For this review, take the finished solid that the model builds, in its own axes (mm). A direction names the side the tool comes from. Give positions to 0.01 mm unless a question says otherwise; leave off trailing zeros. Loops run counter-clockwise (first coordinate to the right, second up) from the corner with the lowest first, then second, coordinate; pieces in that order, holes last. Notation, with made-up numbers: (3, -32) - (15, -32) arc R34 cw to (15, 1) - close; hole circle Ø11 at (49.25, 36.5). An arc over 180 degrees is marked (long way). Put each result on its own line as item: value.
from build123d import *

# Parameters (mm, degrees)
SKETCH1_W                = 60
SKETCH1_H                = 21
BOSS_EXTRUDE1_DEPTH      = 10
BOSS_EXTRUDE1_DEPTH_BACK = 10
FILLET1_R                = 6
SKETCH2_R                = 2.2
CUT_EXTRUDE1_DEPTH       = 21
CUT_EXTRUDE2_DEPTH       = 22


with BuildPart() as part:
    # Sketch1 → Boss-Extrude1 (new body, two sides)
    with BuildSketch(Plane.XY) as boss_extrude1_sk:
        Rectangle(SKETCH1_W, SKETCH1_H)
    extrude(amount=BOSS_EXTRUDE1_DEPTH)
    extrude(boss_extrude1_sk.sketch, amount=-BOSS_EXTRUDE1_DEPTH_BACK)

    # Fillet1
    fillet1_edges = [part.edges().sort_by_distance(p)[0] for p in [
        (30, -10.5, 0),
        (-30, -10.5, 0),
        (-30, 10.5, 0),
        (30, 10.5, 0),
    ]]
    fillet(fillet1_edges, radius=FILLET1_R)

    # Sketch2 → Cut-Extrude1 (cut, through all)
    with BuildSketch(Plane.XY.offset(10)):
        with Locations((-24, 5.5)):
            Circle(SKETCH2_R)
        with Locations((24, 5.5)):
            Circle(SKETCH2_R)
        with Locations((24, -5.5)):
            Circle(SKETCH2_R)
        with Locations((-24, -5.5)):
            Circle(SKETCH2_R)
    extrude(amount=-CUT_EXTRUDE1_DEPTH, mode=Mode.SUBTRACT)

    # Sketch3 → Cut-Extrude2 (cut, through all)
    with BuildSketch(Plane(origin=(0, 10.5, 0), x_dir=(1, 0, 0), z_dir=(0, 1, 0))):
        with BuildLine():
            Line((9, -4.5), (-9, -4.5))
            ThreePointArc((-9, -4.5), (-10.414213562, -3.914213562), (-11, -2.5))
            Line((-11, -2.5), (-11, 2.5))
            ThreePointArc((-11, 2.5), (-10.414213562, 3.914213562), (-9, 4.5))
            Line((-9, 4.5), (9, 4.5))
            ThreePointArc((9, 4.5), (10.414213562, 3.914213562), (11, 2.5))
            Line((11, 2.5), (11, -2.5))
            ThreePointArc((11, -2.5), (10.414213562, -3.914213562), (9, -4.5))
        make_face()
    extrude(amount=-CUT_EXTRUDE2_DEPTH, mode=Mode.SUBTRACT)


solid = part.part
1) Take a section at C-C on z = 8.75. State the section outline as (x, y) points, and give its area (3 significant figures).
Geometry check:
outline: (-30, -4.5) arc R6 ccw to (-24, -10.5) - (24, -10.5) arc R6 ccw to (30, -4.5) - (30, 4.5) arc R6 ccw to (24, 10.5) - (-24, 10.5) arc R6 ccw to (-30, 4.5) - close; hole circle Ø4.4 at (-24, -5.5); hole circle Ø4.4 at (-24, 5.5); hole circle Ø4.4 at (24, -5.5); hole circle Ø4.4 at (24, 5.5)
area: 1,170 mm²
2) Wall thickness on line 1 (Y direction, x = -24, z = 0.75); line 2 (X direction, y = 3.25, z = -2); line 3 (Z direction, x = -0.5, y = -6): over which ranges is each line inside the solid? List them lowest first.
Geometry check:
line 1: y = -10.5 to -7.7, -3.3 to 3.3, 7.7 to 10.5
line 2: x = -30 to -11, 11 to 30
line 3: z = -10 to -4.5, 4.5 to 10
3) Take a section at B-B on y = -5.5. State the section outline as (x, z) points, and give its area (3 significant figures).
Geometry check:
outline: (-29.92, -10) - (-26.2, -10) - (-26.2, 10) - (-29.92, 10) - close; (-21.8, -10) - (21.8, -10) - (21.8, 10) - (-21.8, 10) - close; (26.2, -10) - (29.92, -10) - (29.92, 10) - (26.2, 10) - close; hole (-11, -2.5) arc R2 ccw to (-9, -4.5) - (9, -4.5) arc R2 ccw to (11, -2.5) - (11, 2.5) arc R2 ccw to (9, 4.5) - (-9, 4.5) arc R2 ccw to (-11, 2.5) - close
area: 826 mm²
4) Take a section at D-D on y = -8.75. State the section outline as (x, z) points, and give its area (3 significant figures).
Geometry check:
outline: (-28.24, -10) - (28.24, -10) - (28.24, 10) - (-28.24, 10) - close; hole (-11, -2.5) arc R2 ccw to (-9, -4.5) - (9, -4.5) arc R2 ccw to (11, -2.5) - (11, 2.5) arc R2 ccw to (9, 4.5) - (-9, 4.5) arc R2 ccw to (-11, 2.5) - close
area: 935 mm²
5) For faces 1 (the face through (11, 0, 0)), 2 (the face through (0, 10.5, 5)), list the 3-axis set-ups (+Z, -Z, +X, -X, +Y, -Y) from which the entire face can be reached by the end or side of a thin tool; tool diameter is ignored.
Geometry check:
face 1: +Y, -Y
face 2: +Z, -Z, +X, -X, +Y
6) Take a section at A-A on z = 0.75. State the section outline as (x, y) points.
Geometry check:
outline: (-30, -4.5) arc R6 ccw to (-24, -10.5) - (-11, -10.5) - (-11, 10.5) - (-24, 10.5) arc R6 ccw to (-30, 4.5) - close; (11, -10.5) - (24, -10.5) arc R6 ccw to (30, -4.5) - (30, 4.5) arc R6 ccw to (24, 10.5) - (11, 10.5) - close; hole circle Ø4.4 at (-24, -5.5); hole circle Ø4.4 at (-24, 5.5); hole circle Ø4.4 at (24, -5.5); hole circle Ø4.4 at (24, 5.5)
7) Draft analysis for pull direction Z (two halves, no side actions). For faces 3 (the face through (10.4, 0.15, -3.93)), 4 (the face through (0, 0, 10)), 5 (the face through (28.289, -8.696, 0.14)), state which applies: pulls with the +Z half, pulls with the -Z half, needs draft (parallel to the pull), parting line crosses it, or undercut.
Geometry check:
face 3: undercut
face 4: pulls with the +Z half
face 5: needs draft
